from build123d import *

# Parameters (mm, degrees)
F0_R     = 44.25
F1_DEPTH = 20
F2_R     = 41.25
F3_DEPTH = 17
F4_R     = 1
F5_R     = 8


with BuildPart() as f1:
    # F0 (on Top) → F1 (new body)
    with BuildSketch(Plane.XY):
        Circle(F0_R)
    extrude(amount=F1_DEPTH)

    # F2 (on face) → F3 (cut)
    with BuildSketch(Plane.XY.offset(20)):
        Circle(F2_R)
    extrude(amount=-F3_DEPTH, mode=Mode.SUBTRACT)

    # F4
    f4_edges = [f1.edges().sort_by_distance(p)[0] for p in [
        (-41.25, 0, 3),
    ]]
    fillet(f4_edges, radius=F4_R)

    # F5
    f5_edges = [f1.edges().sort_by_distance(p)[0] for p in [
        (-44.25, 0, 0),
    ]]
    fillet(f5_edges, radius=F5_R)


solid = f1.part
Design review of the part built by this model. Coordinates are the model's own, in mm. Give positions to 0.01 mm unless a question says otherwise; leave off trailing zeros. Write each loop counter-clockwise with the first axis right and the second up, starting at its lowest first coordinate (ties: lowest second). Pieces come first, ordered by that corner, then holes. Notation, with made-up numbers: M -37.75,-34 L 3.25,-34 A37 ccw 3.25,3 Z; hole C 14.25,6 d7. An arc over 180 degrees is marked long. Answer as a JSON object with one key per item and string values. Group by question number.
1) We need section C-C (z = 18.75). Give the boundary of the cut face in (x, y).
2) Mouldability with a two-part tool opening along Y and no side actions: class faces 1 (the face through (-1, 1, 3)), 2 (the face through (-1, 1, 0)), 3 (the face through (-9.59, -43.2, 13.92)), 4 (the face through (-8.94, -40.27, 12.11)) as released by +Y, released by -Y, zero draft, split by the parting line, or undercut.
3) We need section A-A (y = 0). Give the boundary of the cut face in (x, z), and give its area (3 significant figures).
4) For line 1 along Y through (x, z) = (0, 14.75); line 2 along Z through (x, y) = (-5.5, -21.5); line 3 along Y through (x, z) = (13.5, 7.75), list the stretches that pass through material, from the lowest coordinate up.
5) Clearance check with flat-ended pins moving along their axes: pin 1 Ø5 at (x, y) = (8, 26) entering from +Z; pin 2 Ø3 at (x, y) = (30.5, -10) entering from -Z; pin 3 Ø3 at (x, z) = (33.5, 11) entering from +Y; pin 4 Ø8 at (x, z) = (7, 10) entering from +Y. State where each tip first meets the part, or that it passes through.
Answer key:
{
 "1": {"outline": "C 0,0 d88.5; hole C 0,0 d82.5"},
 "2": {"face 1": "undercut", "face 2": "zero draft", "face 3": "split by the parting line", "face 4": "undercut"},
 "3": {"outline": "M -44.25,8 A8 ccw -36.25,0 L 36.25,0 A8 ccw 44.25,8 L 44.25,20 L 41.25,20 L 41.25,4 A1 cw 40.25,3 L -40.25,3 A1 cw -41.25,4 L -41.25,20 L -44.25,20 Z", "area": "340 mm²"},
 "4": {"line 1": "y = -44.25 to -41.25, 41.25 to 44.25", "line 2": "z = 0 to 3", "line 3": "y = -42.14 to -38.98, 38.98 to 42.14"},
 "5": {"pin 1": "stops at z = 3", "pin 2": "stops at z = 0", "pin 3": "stops at y = 30.56", "pin 4": "stops at y = 44.15"}
}
